```python
from build123d import *

# Parameters (mm, degrees)
BOSS_EXTRUDE1_DEPTH = 30
SKETCH2_R           = 4.4
CUT_EXTRUDE1_DEPTH  = 101.775803332
SKETCH4_W           = 26
SKETCH4_H           = 53.255509589
CUT_EXTRUDE2_DEPTH  = 40
CUT_EXTRUDE3_DEPTH  = 13
CUT_EXTRUDE4_DEPTH  = 22
CUT_EXTRUDE5_DEPTH  = 29
CUT_EXTRUDE6_DEPTH  = 13
CUT_EXTRUDE7_DEPTH  = 13
CUT_EXTRUDE8_DEPTH  = 13
CUT_EXTRUDE9_DEPTH  = 13


with BuildPart() as part:
    # Sketch1 → Boss-Extrude1 (new body)
    with BuildSketch(Plane.XY):
        with BuildLine():
            Line((-41.88810428, 5.785), (12.276322136, 15.335649772))
            ThreePointArc((12.276322136, 15.335649772), (27.01721186, 53.031344507), (67.276322136, 57.210252411))
            ThreePointArc((67.276322136, 57.210252411), (70.530137672, 50.676906919), (64.962620823, 45.957301533))
            Line((64.962620823, 45.957301533), (54.969956327, 45.574344273))
            ThreePointArc((54.969956327, 45.574344273), (49.512168838, 43.127692894), (47.276322136, 37.580212676))
            Line((47.276322136, 37.580212676), (47.276322136, 12.580212676))
            ThreePointArc((47.276322136, 12.580212676), (49.033681448, 8.337571989), (53.276322136, 6.580212676))
            Line((53.276322136, 6.580212676), (59.526322136, 6.580212676))
            ThreePointArc((59.526322136, 6.580212676), (74.390705288, -9.127420407), (57.887586742, -23.103353356))
            Line((57.887586742, -23.103353356), (22.023718903, -19.131387173))
            ThreePointArc((22.023718903, -19.131387173), (18.826238067, -18.366578697), (15.915778413, -16.837513523))
            ThreePointArc((15.915778413, -16.837513523), (14.177787103, -15.888509343), (12.276322136, -15.335649772))
            Line((12.276322136, -15.335649772), (-41.88810428, -5.785))
            Line((-41.88810428, -5.785), (-41.88810428, 5.785))
        make_face()
    extrude(amount=BOSS_EXTRUDE1_DEPTH)

    # Sketch2 → Cut-Extrude1 (cut, through all)
    with BuildSketch(Plane.XY.offset(30)):
        with Locations((59.526322136, -8.306805028)):
            Circle(SKETCH2_R)
    extrude(amount=-CUT_EXTRUDE1_DEPTH, mode=Mode.SUBTRACT)

    # Sketch4 → Cut-Extrude2 (cut)
    with BuildSketch(Plane(origin=(70, 0, 0), x_dir=(0, 0, -1), z_dir=(1, 0, 0))):
        with Locations((-15, 24.841006249)):
            Rectangle(SKETCH4_W, SKETCH4_H)
    extrude(amount=-CUT_EXTRUDE2_DEPTH, mode=Mode.SUBTRACT)

    # Sketch5 → Cut-Extrude3 (cut, symmetric)
    with BuildSketch(Plane.XY.offset(15)):
        with BuildLine():
            ThreePointArc((30, 51.468761043), (14.752383127, 23.887752406), (27.160195833, -5.082025668))
            add(Edge.make_bspline(
                [(27.160195833, -5.082025668), (28.094948904, -5.887577241), (30.586732107, -8.19455625), (37.238701336, -9.917559519), (48.959505276, -8.540216128), (58.394612416, -6.238640535), (63.488820328, -1.786748546)],
                knots=[0, 0, 0, 0, 0.09340361, 0.26111983, 0.503691176, 1, 1, 1, 1], degree=3))
            Line((63.488820328, -1.786748546), (35, -1.786748546))
            ThreePointArc((35, -1.786748546), (31.464466094, -0.322282452), (30, 3.213251454))
            Line((30, 3.213251454), (30, 51.468761043))
        make_face()
    extrude(amount=CUT_EXTRUDE3_DEPTH, both=True, mode=Mode.SUBTRACT)

    # Sketch6 → Cut-Extrude4 (cut)
    with BuildSketch(Plane.XY.offset(15)):
        with BuildLine():
            Line((32, 24.594919279), (20, 24.594919279))
            ThreePointArc((20, 24.594919279), (17.878679656, 23.716239623), (17, 21.594919279))
            Line((17, 21.594919279), (17, 15.594919279))
            ThreePointArc((17, 15.594919279), (17.878679656, 13.473598935), (20, 12.594919279))
            Line((20, 12.594919279), (32, 12.594919279))
            ThreePointArc((32, 12.594919279), (34.121320344, 13.473598935), (35, 15.594919279))
            Line((35, 15.594919279), (35, 21.594919279))
            ThreePointArc((35, 21.594919279), (34.121320344, 23.716239623), (32, 24.594919279))
        make_face()
    extrude(amount=-CUT_EXTRUDE4_DEPTH, mode=Mode.SUBTRACT)

    # Sketch7 → Cut-Extrude5 (cut)
    with BuildSketch(Plane.XY.offset(15)):
        with BuildLine():
            Line((28.275, 23.869919279), (23.725, 23.869919279))
            ThreePointArc((23.725, 23.869919279), (21.603679656, 22.991239623), (20.725, 20.869919279))
            Line((20.725, 20.869919279), (20.725, 16.319919279))
            ThreePointArc((20.725, 16.319919279), (21.603679656, 14.198598935), (23.725, 13.319919279))
            Line((23.725, 13.319919279), (28.275, 13.319919279))
            ThreePointArc((28.275, 13.319919279), (30.396320344, 14.198598935), (31.275, 16.319919279))
            Line((31.275, 16.319919279), (31.275, 20.869919279))
            ThreePointArc((31.275, 20.869919279), (30.396320344, 22.991239623), (28.275, 23.869919279))
        make_face()
    extrude(amount=CUT_EXTRUDE5_DEPTH, mode=Mode.SUBTRACT)

    # Sketch9 → Cut-Extrude6 (cut, symmetric)
    with BuildSketch(Plane.XY.offset(15)):
        with BuildLine():
            add(Edge.make_bspline(
                [(27.160195833, -5.082025668), (28.094948904, -5.887577241), (30.586732107, -8.19455625), (37.238701336, -9.917559519), (45.927597, -8.896503874), (52.39349387, -7.580878177), (55.560202392, -6.40157691)],
                knots=[0, 0, 0, 0, 0.09340361, 0.26111983, 0.503691176, 0.765483911, 0.765483911, 0.765483911, 0.765483911], degree=3))
            ThreePointArc((55.560202392, -6.40157691), (61.448410701, -12.264781222), (60.481418473, -4.011715857))
            add(Edge.make_bspline(
                [(60.481418473, -4.011715857), (61.522798548, -3.362828802), (62.527928844, -2.626483629), (63.488820328, -1.786748546)],
                knots=[0.906384087, 0.906384087, 0.906384087, 0.906384087, 1, 1, 1, 1], degree=3))
            Line((63.488820328, -1.786748546), (66.958817178, -1.786748546))
            ThreePointArc((66.958817178, -1.786748546), (68.293766616, -12.876819947), (58.4379775, -18.133738682))
            Line((58.4379775, -18.133738682), (22.574109661, -14.161772498))
            ThreePointArc((22.574109661, -14.161772498), (20.584136694, -13.685788976), (18.772793224, -12.734165333))
            Line((18.772793224, -12.734165333), (22.574109661, -0.326656193))
            Line((22.574109661, -0.326656193), (27.160195833, -5.082025668))
        make_face()
    extrude(amount=CUT_EXTRUDE6_DEPTH, both=True, mode=Mode.SUBTRACT)

    # Sketch10 → Cut-Extrude7 (cut, symmetric)
    with BuildSketch(Plane.XY.offset(15)):
        with BuildLine():
            Line((66.958817178, -1.786748546), (70, -1.786748546))
            Line((70, -1.786748546), (70.49467045, -3.724608486))
            ThreePointArc((70.49467045, -3.724608486), (69.041750074, -15.431257361), (58.217821197, -20.121584551))
            Line((58.217821197, -20.121584551), (22.353953358, -16.149618368))
            ThreePointArc((22.353953358, -16.149618368), (19.880977243, -15.558104864), (17.6299873, -14.375504609))
            Line((17.6299873, -14.375504609), (18.772793224, -12.734165333))
            ThreePointArc((18.772793224, -12.734165333), (20.584136694, -13.685788976), (22.574109661, -14.161772498))
            Line((22.574109661, -14.161772498), (58.4379775, -18.133738682))
            ThreePointArc((58.4379775, -18.133738682), (68.293766616, -12.876819947), (66.958817178, -1.786748546))
        make_face()
    extrude(amount=CUT_EXTRUDE7_DEPTH, both=True, mode=Mode.SUBTRACT)

    # Sketch11 → Cut-Extrude8 (cut, symmetric)
    with BuildSketch(Plane.XY.offset(15)):
        with BuildLine():
            Line((58.217821197, -20.121584551), (57.887586742, -23.103353356))
            ThreePointArc((57.887586742, -23.103353356), (72.259948277, -16.01900714), (71.880280462, 0))
            Line((71.880280462, 0), (70, 0))
            Line((70, 0), (70, -1.786748546))
            Line((70, -1.786748546), (70.49467045, -3.724608486))
            ThreePointArc((70.49467045, -3.724608486), (69.041750074, -15.431257361), (58.217821197, -20.121584551))
        make_face()
    extrude(amount=CUT_EXTRUDE8_DEPTH, both=True, mode=Mode.SUBTRACT)

    # Sketch12 → Cut-Extrude9 (cut, symmetric)
    with BuildSketch(Plane.XY.offset(15)):
        with BuildLine():
            Line((70, 0), (70, 2.272673603))
            ThreePointArc((70, 2.272673603), (70.996566459, 1.183020643), (71.880280462, 0))
            Line((71.880280462, 0), (70, 0))
        make_face()
    extrude(amount=CUT_EXTRUDE9_DEPTH, both=True, mode=Mode.SUBTRACT)


solid = part.part
```
Build history of the part. All positions in model axes, mm. A direction names the side the tool comes from. Round coordinates to 2 decimals unless told otherwise and drop trailing zeros. Loops run counter-clockwise (first coordinate to the right, second up) from the corner with the lowest first, then second, coordinate; pieces in that order, holes last. Notation, with made-up numbers: M 0,84.5 L 17,84.5 A19 ccw 17,99.5 Z; hole C -25,85.5 d1. An arc over 180 degrees is marked long. Answer as CSV lines item,"result".
1. Cut at D-D on x = -20. Write the cut outline in (y, z).
Resolved:
outline,"M -9.64,0 L 9.64,0 L 9.64,30 L -9.64,30 Z"
2. Cut at B-B on y = 4.5. Write the cut outline in (x, z).
Resolved:
outline,"M -41.89,0 L 67.12,0 L 67.12,2 L 19.32,2 L 19.32,28 L 67.12,28 L 67.12,30 L -41.89,30 Z"
3. Cut at A-A on x = 44. Write the cut outline in (y, z).
Resolved:
outline,"M -21.57,0 L 60.42,0 L 60.42,30 L -21.57,30 Z; hole M -18.55,2 L 51.47,2 L 51.47,28 L -18.55,28 Z"
4. Two-plate mould, pull along Z, no slides. Class faces 4 (the flat face through (30, 10, 0)), 5 (the flat face through (-14.427, -10.627, 14.79)), 6 (the flat face through (45, 14, 2)): released by +Z, released by -Z, zero draft, split by the parting line, or undercut.
Resolved:
face 4,"released by -Z"
face 5,"zero draft"
face 6,"undercut"
5. Flat gauge pins, fed straight in: P1, Ø1.6, axis at x = 28.5, z = 1, coming from the +Y side; P2, Ø1, axis at y = 19, z = 1, coming from the +X side; P3, Ø8, axis at y = 15.5, z = 27, coming from the +X side; P4, Ø7, axis at x = 59.53, y = -8.31, coming from the +Z side. Where does each tip first touch, or does it go through?
Resolved:
P1,"stops at y = 54.64"
P2,"stops at x = 47.28"
P3,"stops at x = 47.35"
P4,"passes through"
6. Wall check: probe 1 along Z at (x, y) = (28.5, 9); probe 2 along Y at (x, z) = (52.5, 12); probe 3 along Y at (x, z) = (61, 5). Give the ranges that are in metal, low to high. Write a range as [from, to].
Resolved:
probe 1,"z = [0, 2], [28, 30]"
probe 2,"y = [-22.51, -19.49], [51.47, 60.93]"
probe 3,"y = [51.47, 59.56]"
7. 3-axis set-ups, long thin cutter, end or side, ignore diameter. For faces 1 (the cylindrical face through (30.4, 14.2, 29)), 2 (the cylindrical face through (19.91, -15.57, 15.18)), 3 (the flat face through (70, 50, 15)): which of +Z, -Z, +X, -X, +Y, -Y reach the whole face in a straight line?
Resolved:
face 1,"+Z, -Z"
face 2,"+X"
face 3,"-Y"
